from build123d import *

# Parameters (mm, degrees)
F0_W        = 25
F0_H        = 80
F0_W_2      = 21.83
F0_H_2      = 76.83
F1_DEPTH    = 243.645
F2_T1_DEPTH = 439.0919651514


# Not quite as in the source:
# - a fillet or chamfer that OpenCascade refuses, or shapes differently, is made with other operations: its cross-section is extruded or revolved along the edge and cut away or added


with BuildPart() as f1:
    # F0 (on Front) → F1 (new body, symmetric)
    with BuildSketch(Plane.XZ):
        Rectangle(F0_W, F0_H)
        Rectangle(F0_W_2, F0_H_2, mode=Mode.SUBTRACT)
    extrude(amount=F1_DEPTH, both=True)

    # F2: chamfer of 80 x 43.99 on 1 edges, made by hand

    # F2_s2 → F2_t1 (cut)
    with BuildSketch(Plane.YZ.offset(-219.5459825757)):
        Polygon((-243.645, 40), (-199.655, -40), (-243.645, -40), align=None)
    extrude(amount=F2_T1_DEPTH, mode=Mode.SUBTRACT)


solid = f1.part
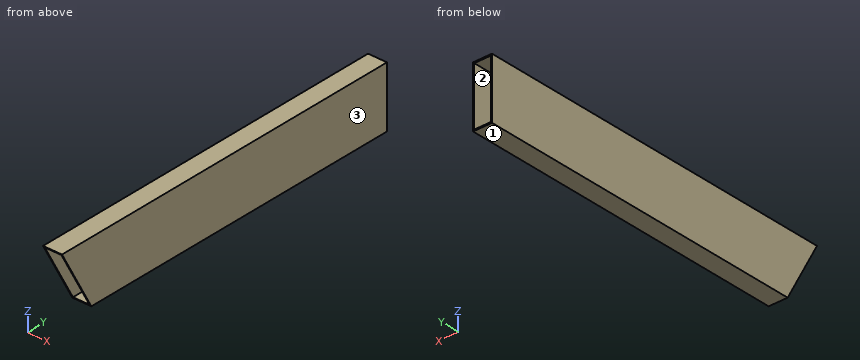
The model under review builds one solid part; all positions refer to its coordinate system, in mm. Face numbers are marked on the shaded views. Give positions to 0.01 mm unless a question says otherwise; leave off trailing zeros. Write each loop counter-clockwise with the first axis right and the second up, starting at its lowest first coordinate (ties: lowest second). Pieces come first, ordered by that corner, then holes. Notation, with made-up numbers: M -2,30 L 38,30 A25 cw 38,51 Z; hole C -30.75,17 d1. An arc over 180 degrees is marked long. One line per question, with ' | ' between items. Start each with the question number.
Item 1: We need section C-C on y = -172. Write out the cut boundary in (x, z) (3 decimals).
Item 2: We need section B-B on z = -2.5. Write out the cut boundary in (x, y) (3 decimals), plus the area to 3 significant figures.
Item 3: Draft analysis for pull direction X (two halves, no side actions). For the marked faces 1, 2 and 3, state which applies: released by +X, released by -X, zero draft, split by the parting line, or undercut.
Item 4: Wall thickness on line 1 (X direction, y = 75, z = -23) (3 decimals); line 2 (Z direction, x = 1, y = -141) (3 decimals): over which ranges is each line inside the solid? List them lowest first. Write a range as from..to.
Item 5: We need section A-A on x = 1. Write out the cut boundary in (y, z) (3 decimals), plus the area to 3 significant figures.
Item 6: For pin 1 (1 mm diameter, centred on x = 10, z = -17, fed in from -Y), flat-tipped, find the tip position at first contact; note if it passes through.
Results found:
1) outline: M -12.5,-40 L 12.5,-40 L 12.5,40 L -12.5,40 Z; hole M -10.915,-38.415 L 10.915,-38.415 L 10.915,38.415 L -10.915,38.415 Z
2) outline: M -12.5,-220.275 L -10.915,-220.275 L -10.915,243.645 L -12.5,243.645 Z; M 10.915,-220.275 L 12.5,-220.275 L 12.5,243.645 L 10.915,243.645 Z | area: 1,470 mm2
3) face 1: zero draft | face 2: undercut | face 3: released by +X
4) line 1: x = -12.5..-10.915, 10.915..12.5 | line 2: z = -40..-38.415, 38.415..40
5) outline: M -243.645,40 L -242.773,38.415 L 243.645,38.415 L 243.645,40 Z; M -200.527,-38.415 L -199.655,-40 L 243.645,-40 L 243.645,-38.415 Z | area: 1,470 mm2
6) pin 1: passes through
